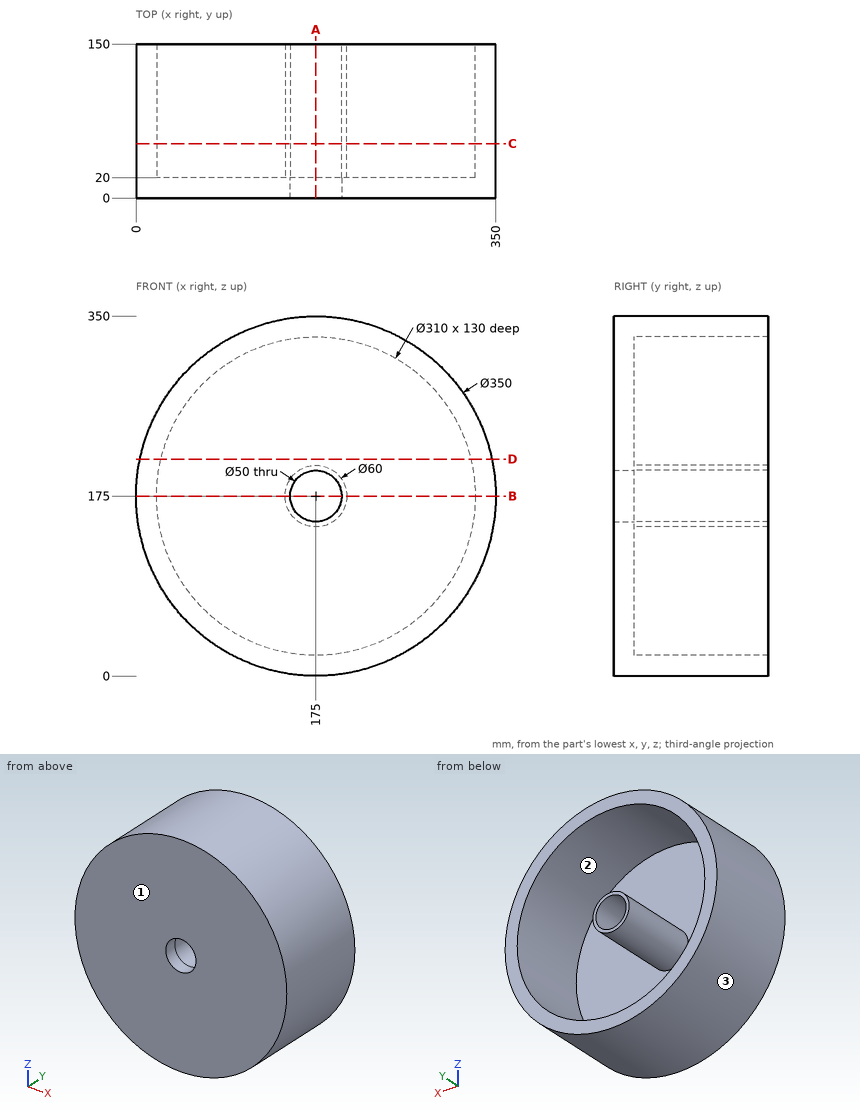
Verification items for this drawing (mm, ordinates from the low corner). Give positions to 0.01 mm unless a question says otherwise; leave off trailing zeros. Loops run counter-clockwise (first coordinate to the right, second up) from the corner with the lowest first, then second, coordinate; pieces in that order, holes last. Notation, with made-up numbers: (-34.5, -2.75) - (-10.5, -2.75) arc R17 cw to (-10.5, 23.25) - close; hole circle Ø3 at (61, -23). An arc over 180 degrees is marked (long way). Write item = value, one per line. Start each with the question number.
Q1. Mould release check, pull along X, two halves, no side actions. Record for the marked faces 1, 2 and 3: released by +X, released by -X, zero draft, split by the parting line, or undercut.
Q2. Cross-section at B-B, the plane z = 175. Enter the section's corners in (x, y).
Q3. Thickness scan on line 1 (X direction, y = 48.5, z = 175); line 2 (X direction, y = 7.5, z = 175). Record the ranges inside material, lowest first.
Q4. Depth check by flat-ended pin: P1, Ø6, axis at y = 127.5, z = 306.5, coming from the +X side; P2, Ø10, axis at y = 90, z = 226.5, coming from the -X side; P3, Ø8, axis at y = 78, z = 87, coming from the -X side. Enter the tip coordinate at first touch or a pass-through.
Q5. Cross-section at A-A, the plane x = 175. Enter the section's corners in (y, z), and give its area (3 significant figures).
Q6. Cross-section at D-D, the plane z = 211. Enter the section's corners in (x, y), and give its area (3 significant figures).
Q7. Cross-section at C-C, the plane y = 53. Enter the section's corners in (x, z), and give its area (3 significant figures).
Answer key:
q1.face_1 = zero draft
q1.face_2 = undercut
q1.face_3 = split by the parting line
q2.outline = (0, 0) - (150, 0) - (150, 150) - (145, 150) - (145, 20) - (20, 20) - (20, 150) - (0, 150) - close; (200, 0) - (350, 0) - (350, 150) - (330, 150) - (330, 20) - (205, 20) - (205, 150) - (200, 150) - close
q3.line_1 = 0 to 20, 145 to 150, 200 to 205, 330 to 350
q3.line_2 = 0 to 150, 200 to 350
q4.P1 = 293.8
q4.P2 = 6.29
q4.P3 = 21.48
q5.outline = (0, 0) - (150, 0) - (150, 20) - (20, 20) - (20, 145) - (150, 145) - (150, 150) - (0, 150) - close; (0, 200) - (150, 200) - (150, 205) - (20, 205) - (20, 330) - (150, 330) - (150, 350) - (0, 350) - close
q5.area = 12,500 mm^2
q6.outline = (3.74, 0) - (346.26, 0) - (346.26, 150) - (325.76, 150) - (325.76, 20) - (24.24, 20) - (24.24, 150) - (3.74, 150) - close
q6.area = 12,200 mm^2
q7.outline = circle Ø350 at (175, 175); circle Ø60 at (175, 175); hole circle Ø310 at (175, 175); hole circle Ø50 at (175, 175)
q7.area = 21,600 mm^2
